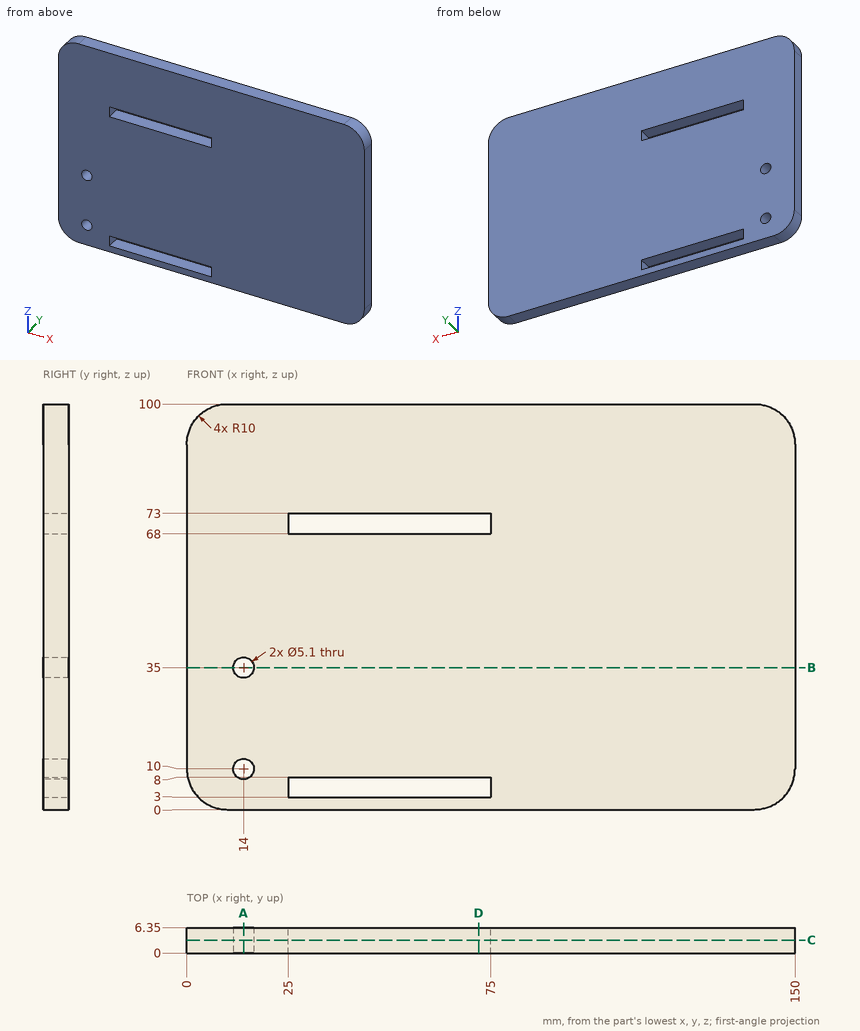
Check sheet for the drawn part. Datum: minimum x, y, z corner. Units: mm. Round coordinates to 2 decimals unless told otherwise and drop trailing zeros. Order: outer loops, then holes, each group sorted by start corner. A loop starts at its lowest first (then second) coordinate and runs counter-clockwise, first axis right, second up. Notation, with made-up numbers: (78, -13) -> (108, -13) arc R15 cw to (108, -7) -> close; hole circle Ø6 at (25.25, 49). An arc over 180 degrees is marked (long way). Use CSV: the item, a comma, the result in double quotes.
(1) Cross-section at D-D (x = 72). Record the boundary of the cut face in (y, z).
Worked out:
outline,"(0, 0) -> (6.35, 0) -> (6.35, 3) -> (0, 3) -> close; (0, 8) -> (6.35, 8) -> (6.35, 68) -> (0, 68) -> close; (0, 73) -> (6.35, 73) -> (6.35, 100) -> (0, 100) -> close"
(2) Depth check by flat-ended pin: pin 1 (1.5 mm diameter, centred on y = 3.5, z = 5, fed in from -X); pin 2 (4 mm diameter, centred on x = 14, z = 10, fed in from -Y). Enter the tip coordinate at first touch or a pass-through.
Worked out:
pin 1,"x = 0.95"
pin 2,"through"
(3) Cross-section at B-B (z = 35). Record the boundary of the cut face in (x, y), and give its area (3 significant figures).
Worked out:
outline,"(0, 0) -> (11.45, 0) -> (11.45, 6.35) -> (0, 6.35) -> close; (16.55, 0) -> (150, 0) -> (150, 6.35) -> (16.55, 6.35) -> close"
area,"920 mm²"
(4) Cross-section at A-A (x = 14). Record the boundary of the cut face in (y, z).
Worked out:
outline,"(0, 0) -> (6.35, 0) -> (6.35, 7.45) -> (0, 7.45) -> close; (0, 12.55) -> (6.35, 12.55) -> (6.35, 32.45) -> (0, 32.45) -> close; (0, 37.55) -> (6.35, 37.55) -> (6.35, 100) -> (0, 100) -> close"
(5) Cross-section at C-C (y = 3.25). Record the boundary of the cut face in (x, z), and give its area (3 significant figures).
Worked out:
outline,"(0, 10) arc R10 ccw to (10, 0) -> (140, 0) arc R10 ccw to (150, 10) -> (150, 90) arc R10 ccw to (140, 100) -> (10, 100) arc R10 ccw to (0, 90) -> close; hole circle Ø5.1 at (14, 10); hole circle Ø5.1 at (14, 35); hole (25, 3) -> (75, 3) -> (75, 8) -> (25, 8) -> close; hole (25, 68) -> (75, 68) -> (75, 73) -> (25, 73) -> close"
area,"14,400 mm²"
(6) Material ranges on line 1 along X through (y, z) = (1.5, 10); line 2 along X through (y, z) = (3, 4); line 3 along Z through (x, y) = (7, 2), recorded low to high. Write a range as from..to.
Worked out:
line 1,"0..11.45, 16.55..150"
line 2,"2..25, 75..148"
line 3,"0.46..99.54"
